from build123d import *

# Parameters (mm, degrees)
BOSS_EXTRUDE1_DEPTH      = 38.1
BOSS_EXTRUDE1_DEPTH_BACK = 312.42
SKETCH1_R                = 3.175
BOSS_EXTRUDE2_DEPTH      = 12.7
SKETCH6_R                = 6.35
BOSS_EXTRUDE3_DEPTH      = 12.7
BOSS_EXTRUDE3_DRAFT      = -15
SKETCH7_R                = 26.162
CUT_EXTRUDE1_DEPTH       = 31.75
FILLET1_R                = 2.54


with BuildPart() as part:
    # Sketch1 → Boss-Extrude1 (new, two sides: drawn at the far end of the back side and taken through both)
    with BuildSketch(Plane.XY.offset(-BOSS_EXTRUDE1_DEPTH_BACK)):
        Circle(SKETCH1_R)
    extrude(amount=BOSS_EXTRUDE1_DEPTH + BOSS_EXTRUDE1_DEPTH_BACK)

    # Sketch5 → Boss-Extrude2 (add)
    with BuildSketch(Plane.XY.offset(38.1)):
        with BuildLine():
            Line((0, -3.181219399), (-50.403125, -6.337585521))
            ThreePointArc((-50.403125, -6.337585521), (-57.15, 0), (-50.403125, 6.337585521))
            Line((-50.403125, 6.337585521), (0, 3.181219399))
            ThreePointArc((0, 3.181219399), (3.181219399, 0), (0, -3.181219399))
        make_face()
    extrude(amount=BOSS_EXTRUDE2_DEPTH)


with BuildPart() as boss_extrude3_tool:
    # Sketch6 → Boss-Extrude3 (with draft: the straight prism first)
    with BuildSketch(Plane.XY.offset(50.8)):
        with Locations((-50.8, 0)):
            Circle(SKETCH6_R)
    extrude(amount=BOSS_EXTRUDE3_DEPTH)
    # Boss-Extrude3: the draft: its side faces are tilted about the plane it starts from
    boss_extrude3_sides = [boss_extrude3_tool.faces().sort_by_distance(p)[0] for p in [
        (-57.15, 0, 57.15),
    ]]
    draft(boss_extrude3_sides, Plane.XY.offset(50.8), BOSS_EXTRUDE3_DRAFT)


with BuildPart() as part_1:
    add(part.part)

    # Boss-Extrude3: add boss_extrude3_tool
    add(boss_extrude3_tool.part)

    # Sketch7 → Cut-Extrude1 (cut)
    with BuildSketch(Plane(origin=(0, 0, -312.42), x_dir=(-1, 0, 0), z_dir=(0, 0, -1))):
        Circle(SKETCH7_R)
    extrude(amount=-CUT_EXTRUDE1_DEPTH, mode=Mode.SUBTRACT)

    # Fillet1
    fillet1_edges = [part_1.edges().sort_by_distance(p)[0] for p in [
        (-60.552954744, 0, 63.5),
    ]]
    fillet(fillet1_edges, radius=FILLET1_R)


solid = part_1.part
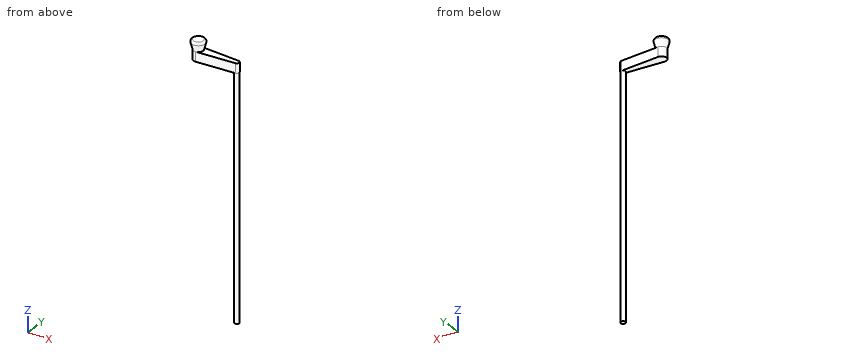
Work out the finished part from the listing and answer in its coordinate system (mm). Give positions to 0.01 mm unless a question says otherwise; leave off trailing zeros. Loops run counter-clockwise (first coordinate to the right, second up) from the corner with the lowest first, then second, coordinate; pieces in that order, holes last. Notation, with made-up numbers: (59.25, 59) - (65.25, 59) arc R15 ccw to (65.25, 78) - close; hole circle Ø4 at (61.25, -10.75). An arc over 180 degrees is marked (long way). Answer in a Markdown table with one row per item.
(1) Consider L1, parallel to Z at x = -36.5, y = -1.75; L2, parallel to X at y = 0, z = 12.5 (3 decimals); L3, parallel to Z at x = -55, y = 3.25. Determine where each line is inside the solid, lowest interval first. Write a range as [from, to].
Results list:
| item | result |
|---|---|
| L1 | z = [38.1, 50.8] |
| L2 | x = [-3.175, 3.175] |
| L3 | z = [38.1, 63.5] |
(2) Section D-D (x = -39) is taken. Give the vertices of the cut face in (y, z).
Results list:
| item | result |
|---|---|
| outline | (-5.62, 38.1) - (5.62, 38.1) - (5.62, 50.8) - (-5.62, 50.8) - close |
(3) Section A-A (y = 0) is taken. Give the vertices of the cut face in (x, z) (3 decimals), and give its area (3 significant figures).
Results list:
| item | result |
|---|---|
| outline | (-59.696, 60.303) - (-57.15, 50.8) - (-57.15, 38.1) - (-3.175, 38.1) - (-3.175, -280.67) - (3.175, -280.67) - (3.175, 38.1) - (3.181, 38.1) - (3.181, 50.8) - (-44.45, 50.8) - (-41.904, 60.303) arc R2.54 ccw to (-44.357, 63.5) - (-57.243, 63.5) arc R2.54 ccw to start |
| area | 2,990 mm² |
(4) Section C-C (x = -20.5) is taken. Give the vertices of the cut face in (y, z).
Results list:
| item | result |
|---|---|
| outline | (-4.46, 38.1) - (4.46, 38.1) - (4.46, 50.8) - (-4.46, 50.8) - close |
(5) Flat-ended cylindrical pins translate along their axes: pin 1 Ø5 at (y, z) = (-3, -41.5) entering from -X; pin 2 Ø10 at (y, z) = (5, 21.5) entering from -X (3 decimals); pin 3 Ø5 at (x, y) = (-28, -4.5) entering from +Z. Find the tip coordinate at first contact, or state that the pin passes through.
Results list:
| item | result |
|---|---|
| pin 1 | stops at x = -3.14 |
| pin 2 | stops at x = -3.175 |
| pin 3 | stops at z = 50.8 |
(6) Section B-B (z = -254.5) is taken. Give the vertices of the cut face in (x, y) (3 decimals), and give its area (3 significant figures).
Results list:
| item | result |
|---|---|
| outline | circle Ø6.35 at (0, 0) |
| area | 31.7 mm² |
